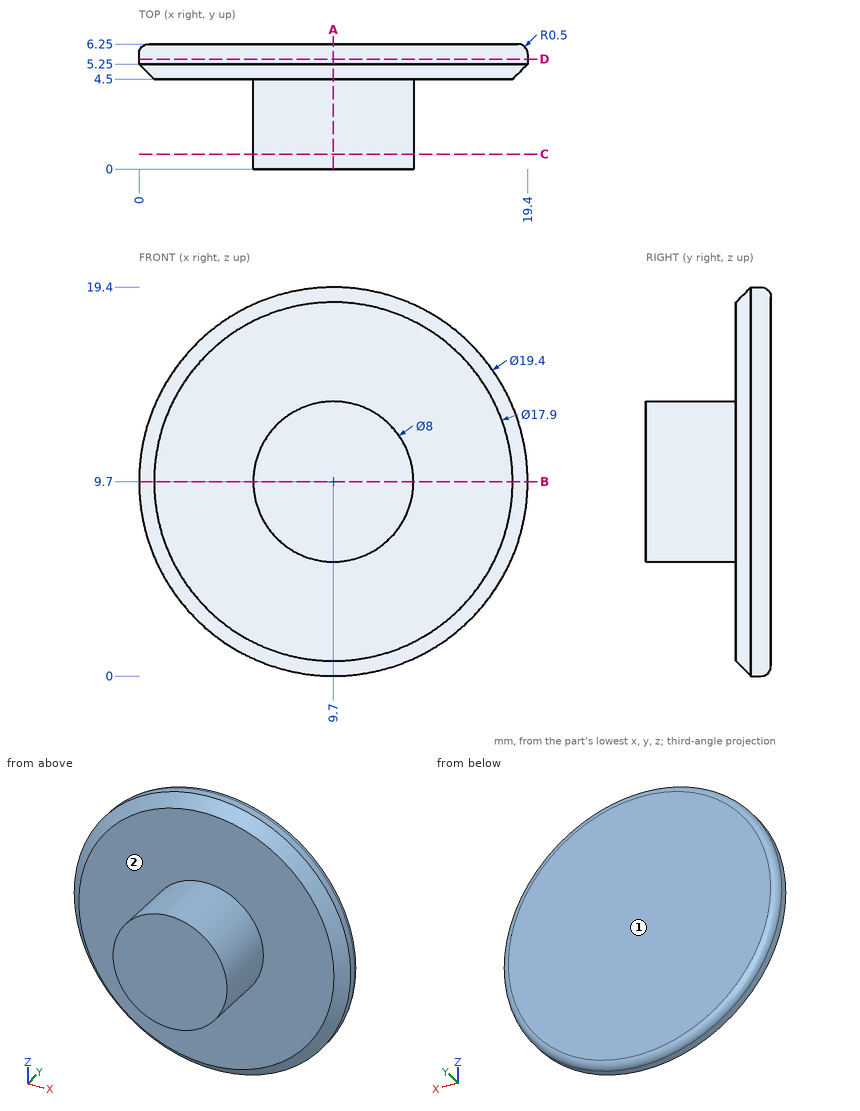
Study the drawing (mm; zero at the part's minimum x, y, z) and answer. A direction names the side the tool comes from. Round coordinates to 2 decimals unless told otherwise and drop trailing zeros. Write each loop counter-clockwise with the first axis right and the second up, starting at its lowest first coordinate (ties: lowest second). Pieces come first, ordered by that corner, then holes. Notation, with made-up numbers: (84, 58) - (100, 58) arc R14 cw to (100, 70) - close; hole circle Ø4 at (86, 11.25). An arc over 180 degrees is marked (long way). Return JSON: item names as keys, results as strings. Group by question number.
Q1. The part is cut by section B-B on z = 9.7. Write down the section's boundary in (x, y), then the cut area to 3 significant figures.
Q2. For the marked faces 1 and 2, determine the directions among +Z, -Z, +X, -X, +Y, -Y from which every point of the face is accessible in a straight line to the end or side of a thin tool.
Q3. The part is cut by section C-C on y = 0.75. Write down the section's boundary in (x, z), then the cut area to 3 significant figures.
Q4. The part is cut by section D-D on y = 5.5. Write down the section's boundary in (x, z), then the cut area to 3 significant figures.
Q5. Find the intervals of material crossed by L1, parallel to Y at x = 3.5, z = 14.75; L2, parallel to Z at x = 16.75, y = 5.75; L3, parallel to Z at x = 13.25, y = 6, in increasing order.
Q6. The part is cut by section A-A on x = 9.7. Write down the section's boundary in (y, z).
Q7. Each of these flat-tipped pins is pushed along its axis until it touches: pin 1 Ø1 at (x, y) = (5, 5.5) entering from -Z; pin 2 Ø2 at (x, y) = (5, 4) entering from -Z; pin 3 Ø4 at (x, z) = (4, 7.5) entering from -Y. Where does it stop, or does it pass through?
Solved:
{
 "1": {"outline": "(0, 5.25) - (0.75, 4.5) - (5.7, 4.5) - (5.7, 0) - (13.7, 0) - (13.7, 4.5) - (18.65, 4.5) - (19.4, 5.25) - (19.4, 5.75) arc R0.5 ccw to (18.9, 6.25) - (0.5, 6.25) arc R0.5 ccw to (0, 5.75) - close", "area": "69.3 mm²"},
 "2": {"face 1": "+Z, -Z, +X, -X, +Y", "face 2": "-Y"},
 "3": {"outline": "circle Ø8 at (9.7, 9.7)", "area": "50.3 mm²"},
 "4": {"outline": "circle Ø19.4 at (9.7, 9.7)", "area": "296 mm²"},
 "5": {"L1": "4.5 to 6.25", "L2": "3.04 to 16.36", "L3": "0.74 to 18.66"},
 "6": {"outline": "(0, 5.7) - (4.5, 5.7) - (4.5, 0.75) - (5.25, 0) - (5.75, 0) arc R0.5 ccw to (6.25, 0.5) - (6.25, 18.9) arc R0.5 ccw to (5.75, 19.4) - (5.25, 19.4) - (4.5, 18.65) - (4.5, 13.7) - (0, 13.7) - close"},
 "7": {"pin 1": "z = 0.96", "pin 2": "z = 1.38", "pin 3": "y = 4.5"}
}
